CAD build for the part. Positions are in the model's coordinates, mm. A direction names the side the tool comes from. Coordinates: 2 decimals unless noted, no trailing zeros. Order: outer loops, then holes, each group sorted by start corner. A loop starts at its lowest first (then second) coordinate and runs counter-clockwise, first axis right, second up. Notation, with made-up numbers: (-32, 35.25) - (21, 35.25) arc R19 cw to (21, 56.25) - close; hole circle Ø2 at (-23, 69.25). An arc over 180 degrees is marked (long way). Return JSON: item names as keys, results as strings.
Autodesk Inventor part; units mm, degrees
ref_plane "YZ Plane" through (0, 0, 0) normal (1, 0, 0) x (0, 1, 0)
ref_plane "XZ Plane" through (0, 0, 0) normal (0, 1, 0) x (-1, 0, 0)
ref_plane "XY Plane" through (0, 0, 0) normal (0, 0, 1) x (1, 0, 0)
sketch "Sketch1" plane through (0, 0, 0) normal (1, 0, 0) x (0, 1, 0)
  line L0 (-25, -25) -> (25, -25)
  line L1 (25, -25) -> (25, 25)
  line L2 (25, 25) -> (-25, 25)
  line L3 (-25, 25) -> (-25, -25)
  line L4 (-25, -25) -> (25, 25) construction
  line L5 (25, -25) -> (-25, 25) construction
  line L6 (-24, -24) -> (24, -24)
  line L7 (24, -24) -> (24, 24)
  line L8 (24, 24) -> (-24, 24)
  line L9 (-24, 24) -> (-24, -24)
  line L10 (-24, -24) -> (24, 24) construction
  line L11 (24, -24) -> (-24, 24) construction
  point P0 (0, 0)
  dimension "d0" = 50
  dimension "d1" = 50
  dimension "d2" = 48
  dimension "d3" = 48
extrude "Extrusion1" add sketch "Sketch1" along normal blind 2 contours L3 L2 L1 L0 | L9 L8 L7 L6
sketch "Sketch3" plane through (0, 0, 0) normal (-1, 0, 0) x (0, 0, 1)
  line L0 (19.3, -19.3) -> (-19.3, -19.3)
  line L1 (-19.3, -19.3) -> (-19.3, 19.3)
  line L2 (-19.3, 19.3) -> (19.3, 19.3)
  line L3 (19.3, 19.3) -> (19.3, -19.3)
  line L4 (19.3, -19.3) -> (-19.3, 19.3) construction
  line L5 (-19.3, -19.3) -> (19.3, 19.3) construction
  circle A0 centre (-19.3, 19.3) radius 1.5
  circle A1 centre (19.3, 19.3) radius 1.5555
  circle A2 centre (19.3, -19.3) radius 1.5555
  circle A3 centre (-19.3, -19.3) radius 1.5555
  point P0 (0, 0)
  dimension "d6" = 38.6
  dimension "d7" = 38.6
  dimension "d8" = 3
  dimension "d9" = 3.111
  dimension "d10" = 3.111
  dimension "d11" = 3.111
hole "Hole1" at (0, 19.3, -19.3) direction (1, 0, 0) diameter 3 end through all
sketch "Sketch4" plane through (0, 0, 0) normal (-1, 0, 0) x (0, 0, 1)
  line L0 (-19.3, -19.3) -> (19.3, -19.3)
  line L1 (19.3, -19.3) -> (19.3, 19.3)
  line L2 (19.3, 19.3) -> (-19.3, 19.3)
  line L3 (-19.3, 19.3) -> (-19.3, -19.3)
  line L4 (-19.3, -19.3) -> (19.3, 19.3) construction
  line L5 (19.3, -19.3) -> (-19.3, 19.3) construction
  circle A0 centre (19.3, 19.3) radius 1.5
  point P0 (0, 0)
  dimension "d19" = 38.6
  dimension "d20" = 38.6
  dimension "d21" = 3
hole "Hole2" at (0, 19.3, 19.3) direction (1, 0, 0) diameter 3 end through all
sketch "Sketch5" plane through (0, 0, 0) normal (-1, 0, 0) x (0, 0, 1)
  line L0 (19.3, -19.3) -> (-19.3, -19.3)
  line L1 (-19.3, -19.3) -> (-19.3, 19.3)
  line L2 (-19.3, 19.3) -> (19.3, 19.3)
  line L3 (19.3, 19.3) -> (19.3, -19.3)
  line L4 (19.3, -19.3) -> (-19.3, 19.3) construction
  line L5 (-19.3, -19.3) -> (19.3, 19.3) construction
  circle A0 centre (-19.3, -19.3) radius 1.5
  point P0 (0, 0)
  dimension "d29" = 38.6
  dimension "d30" = 38.6
  dimension "d31" = 3
hole "Hole3" at (0, -19.3, -19.3) direction (1, 0, 0) diameter 3 end through all
sketch "Sketch6" plane through (0, 0, 0) normal (-1, 0, 0) x (0, 0, 1)
  line L0 (19.3, -19.3) -> (-19.3, -19.3)
  line L1 (-19.3, -19.3) -> (-19.3, 19.3)
  line L2 (-19.3, 19.3) -> (19.3, 19.3)
  line L3 (19.3, 19.3) -> (19.3, -19.3)
  line L4 (19.3, -19.3) -> (-19.3, 19.3) construction
  line L5 (-19.3, -19.3) -> (19.3, 19.3) construction
  circle A0 centre (19.3, -19.3) radius 1.5
  point P0 (0, 0)
  dimension "d39" = 38.6
  dimension "d40" = 38.6
  dimension "d41" = 3
hole "Hole4" at (0, -19.3, 19.3) direction (1, 0, 0) diameter 3 end through all
sketch "Sketch7" plane through (0, 0, 0) normal (-1, 0, 0) x (0, 0, 1)
  line L0 (23, -23) -> (-23, -23)
  line L1 (-23, -23) -> (-23, 23)
  line L2 (-23, 23) -> (23, 23)
  line L3 (23, 23) -> (23, -23)
  line L4 (23, -23) -> (-23, 23) construction
  line L5 (-23, -23) -> (23, 23) construction
  line L6 (-25, 25) -> (25, 25)
  line L7 (10, 21) -> (-10, 21)
  line L8 (-10, 21) -> (-10, 25)
  line L9 (-10, 25) -> (10, 25)
  line L10 (10, 25) -> (10, 21)
  line L11 (10, 21) -> (-10, 25) construction
  line L12 (-10, 21) -> (10, 25) construction
  line L13 (21, -10) -> (25, -10)
  line L14 (25, -10) -> (25, 10)
  line L15 (25, 10) -> (21, 10)
  line L16 (21, 10) -> (21, -10)
  line L17 (21, -10) -> (25, 10) construction
  line L18 (25, -10) -> (21, 10) construction
  line L19 (25, -25) -> (-25, -25)
  line L20 (-10, -21) -> (10, -21)
  line L21 (10, -21) -> (10, -25)
  line L22 (10, -25) -> (-10, -25)
  line L23 (-10, -25) -> (-10, -21)
  line L24 (-10, -21) -> (10, -25) construction
  line L25 (10, -21) -> (-10, -25) construction
  line L26 (-25.0252, 10) -> (-20.9748, 10)
  line L27 (-20.9748, 10) -> (-20.9748, -10)
  line L28 (-20.9748, -10) -> (-25.0252, -10)
  line L29 (-25.0252, -10) -> (-25.0252, 10)
  line L30 (-25.0252, 10) -> (-20.9748, -10) construction
  line L31 (-20.9748, 10) -> (-25.0252, -10) construction
  line L32 (25, -25) -> (-25, -25)
  line L33 (-25, -25) -> (-25, 25)
  line L34 (-25, 25) -> (25, 25)
  line L35 (25, 25) -> (25, -25)
  line L36 (25, -25) -> (-25, 25) construction
  line L37 (-25, -25) -> (25, 25) construction
  point P0 (0, 0)
  point P1 (0, 23)
  point P2 (23, 0)
  point P3 (0, -23)
  point P4 (-23, 0)
  point P5 (-10, 23)
  point P6 (10, 23)
  point P7 (23, 10)
  point P8 (23, -10)
  point P9 (10, -23)
  point P10 (-10, -23)
  point P11 (-23, -10)
  point P12 (-23, 10)
  point P13 (10, 25)
  point P14 (-25, 10)
  point P15 (-25, -10)
  point P16 (-10, -25)
  dimension "d49" = 46
  dimension "d50" = 46
  dimension "d51" = 20
  dimension "d52" = 20
  dimension "d53" = 20
  dimension "d54" = 20
extrude "Extrusion3" cut sketch "Sketch7" against normal blind 2 contours L3 L13 L35 L19 L21 L0 | L23 L19 L33 L28 L1 L0 | L3 L2 L10 L6 L35 L15 | L26 L33 L6 L8 L2 L1
sketch "Sketch8" plane through (2, 0, 0) normal (1, 0, 0) x (0, 0, -1)
  circle A0 centre (0, 0) radius 9
  dimension "d59" = 18
extrude "Extrusion4" cut sketch "Sketch8" against normal blind 2
sketch "Sketch9" plane through (2, 0, 0) normal (1, 0, 0) x (0, 0, -1)
  line L0 (13.75, -13.75) -> (-13.75, -13.75)
  line L1 (-13.75, -13.75) -> (-13.75, 13.75)
  line L2 (-13.75, 13.75) -> (13.75, 13.75)
  line L3 (13.75, 13.75) -> (13.75, -13.75)
  line L4 (13.75, -13.75) -> (-13.75, 13.75) construction
  line L5 (-13.75, -13.75) -> (13.75, 13.75) construction
  circle A0 centre (-13.75, 13.75) radius 1
  circle A1 centre (13.75, 13.75) radius 1
  circle A2 centre (13.75, -13.75) radius 1
  circle A3 centre (-13.75, -13.75) radius 1
  point P0 (0, 0)
  dimension "d62" = 27.5
  dimension "d63" = 27.5
  dimension "d64" = 2
  dimension "d65" = 2
  dimension "d66" = 2
  dimension "d67" = 2
extrude "Extrusion5" [suppressed]
fillet "Fillet1" radius 2 4 edges at (1, 23, 23) (1, -23, 23) (1, -23, -23) (1, 23, -23)
properties part number "UpperSide" material "Aluminum 6061, Welded"
Item 1: Band-saw the part on B-B, the plane y = -19.3. List the corners of the cut face in (x, z), then the cut area to 3 significant figures.
Findings below:
{"outline": "(0, -23) - (2, -23) - (2, -20.8) - (0, -20.8) - close; (0, -17.8) - (2, -17.8) - (2, 17.8) - (0, 17.8) - close; (0, 20.8) - (2, 20.8) - (2, 23) - (0, 23) - close", "area": "80.0 mm²"}
Item 2: Wall check: L1, parallel to Z at x = 0.65, y = 19.3; L2, parallel to Y at x = 1.3, z = 0. Give the ranges that are in metal, low to high. Write a range as [from, to].
Findings below:
{"L1": "z = [-23, -20.8], [-17.8, 17.8], [20.8, 23]", "L2": "y = [-25, -9], [9, 25]"}
Item 3: Band-saw the part on D-D, the plane x = 0.5. Count the separate pieces of the cut face and the enclosed holes in it, then the cut area to 3 significant figures.
Findings below:
{"separate pieces": "1", "enclosed holes": "5", "area": "1,990 mm²"}
Item 4: Which spindle directions (+Z, -Z, +X, -X, +Y, -Y) get a long thin tool onto all of the face, cutting with end or side? Do faces 4 (the flat face through (1, -24, 10)), 5 (the flat face through (1, 16, 23)), 6 (the flat face through (1, 10, -24)). Say none if no direction does.
Findings below:
{"face 4": "+Z, +X, -X, -Y", "face 5": "+Z, +X, -X, +Y", "face 6": "-Z, +X, -X, +Y"}
Item 5: Band-saw the part on A-A, the plane z = 0. List the corners of the cut face in (x, y).
Findings below:
{"outline": "(0, -25) - (2, -25) - (2, -9) - (0, -9) - close; (0, 9) - (2, 9) - (2, 25) - (0, 25) - close"}
Item 6: Drop flat-ended pins along their axis: P1, Ø0.6, axis at x = 0.5, y = 23.5, coming from the -Z side; P2, Ø0.6, axis at x = 1.5, y = -18, coming from the -Z side; P3, Ø2.5, axis at y = -19.3, z = -19.3, coming from the +X side; P4, Ø0.6, axis at x = 0.5, z = 24.5, coming from the -Y side. Give the stop position or say it passes through.
Findings below:
{"P1": "stops at z = -10", "P2": "stops at z = -23", "P3": "passes through", "P4": "stops at y = -10"}
Item 7: Mould opens along Y. For faces 1 (the cylindrical face through (1.014, 18.035, -18.494)), 2 (the flat face through (0, 11, 0)), 3 (the cylindrical face through (1.01, 22.43, 22.4)) say: released by +Y, released by -Y, zero draft, split by the parting line, or undercut.
Findings below:
{"face 1": "undercut", "face 2": "zero draft", "face 3": "released by +Y"}
